The figure shows three views and two pictorial views of one solid part (mm, origin at its lowest corner). Answer the questions. A direction names the side the tool comes from. Give positions to 0.01 mm unless a question says otherwise; leave off trailing zeros. Loops run counter-clockwise (first coordinate to the right, second up) from the corner with the lowest first, then second, coordinate; pieces in that order, holes last. Notation, with made-up numbers: (10, 7.5) -> (65, 7.5) arc R3 ccw to (65, 11.5) -> close; hole circle Ø1 at (71, -15). An arc over 180 degrees is marked (long way). One line per item, written item: value. Start each with the question number.
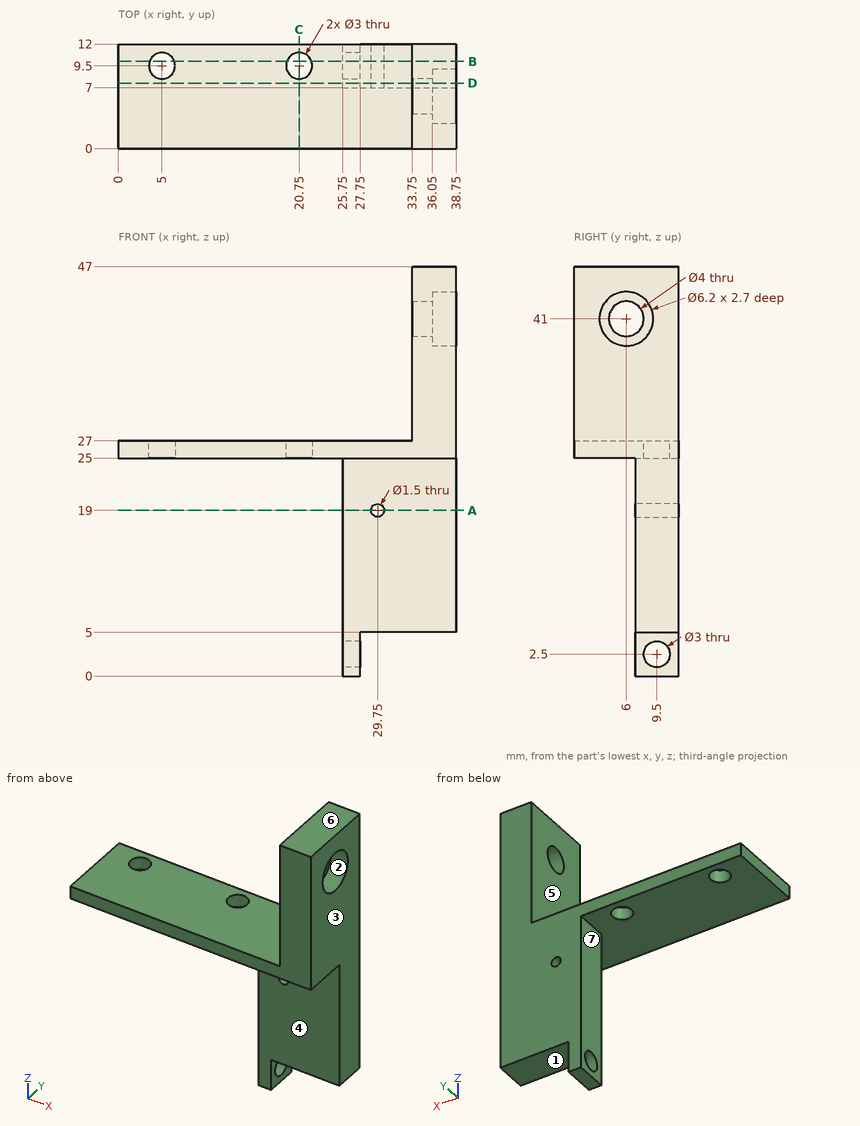
Item 1: Flat-ended cylindrical pins translate along their axes: pin 1 (2.5 mm diameter, centred on x = 29.75, z = 19, fed in from -Y); pin 2 (12 mm diameter, centred on x = 21.5, z = 38, fed in from -Y); pin 3 (1.5 mm diameter, centred on y = 10, z = 1.5, fed in from +X); pin 4 (1.5 mm diameter, centred on y = 9, z = 11, fed in from -X). Find the tip coordinate at first contact, or state that the pin passes through.
Item 2: For the marked faces 4, 5, 6 and 7, determine the directions among +Z, -Z, +X, -X, +Y, -Y from which every point of the face is accessible in a straight line to the end or side of a thin tool.
Item 3: Section D-D, the plane y = 7.5 is taken. Determine the outline of the cut face in (x, z), plus the area to 3 significant figures.
Item 4: Determine the mould class of the marked faces 1, 2 and 3 for opening direction Z: pulls with the +Z half, pulls with the -Z half, needs draft (parallel to the pull), parting line crosses it, or undercut.
Item 5: Consider L1, parallel to X at y = 10.8, z = 19; L2, parallel to Z at x = 37.6, y = 6; L3, parallel to Z at x = 22.5, y = 4.75. Determine where each line is inside the solid, lowest interval first. Write a range as [from, to].
Item 6: Section C-C, the plane x = 20.75 is taken. Determine the outline of the cut face in (y, z).
Item 7: Section A-A, the plane z = 19 is taken. Determine the outline of the cut face in (x, y), plus the area to 3 significant figures.
Item 8: Section B-B, the plane y = 10 is taken. Determine the outline of the cut face in (x, z), plus the area to 3 significant figures.
Computed values:
1. pin 1: y = 7
1. pin 2: through
1. pin 3: x = 27.75
1. pin 4: x = 25.75
2. face 4: -Z, +X, -X, -Y
2. face 5: +Z, -X, +Y, -Y
2. face 6: +Z, +X, -X, +Y, -Y
2. face 7: -Z, -X, +Y, -Y
3. outline: (0, 25) -> (25.75, 25) -> (25.75, 0) -> (27.75, 0) -> (27.75, 5) -> (38.75, 5) -> (38.75, 38.29) -> (36.05, 38.29) -> (36.05, 39.68) -> (33.75, 39.68) -> (33.75, 27) -> (0, 27) -> close; (33.75, 42.32) -> (36.05, 42.32) -> (36.05, 43.71) -> (38.75, 43.71) -> (38.75, 47) -> (33.75, 47) -> close; hole circle Ø1.5 at (29.75, 19)
3. area: 425 mm²
4. face 1: pulls with the -Z half
4. face 2: undercut
4. face 3: needs draft
5. L1: [25.75, 29], [30.5, 38.75]
5. L2: [25, 37.9], [44.1, 47]
5. L3: [25, 27]
6. outline: (0, 25) -> (8, 25) -> (8, 27) -> (0, 27) -> close; (11, 25) -> (12, 25) -> (12, 27) -> (11, 27) -> close
7. outline: (25.75, 7) -> (29, 7) -> (29, 12) -> (25.75, 12) -> close; (30.5, 7) -> (38.75, 7) -> (38.75, 12) -> (30.5, 12) -> close
7. area: 57.5 mm²
8. outline: (0, 25) -> (3.59, 25) -> (3.59, 27) -> (0, 27) -> close; (6.41, 25) -> (19.34, 25) -> (19.34, 27) -> (6.41, 27) -> close; (22.16, 25) -> (25.75, 25) -> (25.75, 3.91) -> (27.75, 3.91) -> (27.75, 5) -> (38.75, 5) -> (38.75, 47) -> (33.75, 47) -> (33.75, 27) -> (22.16, 27) -> close; (25.75, 0) -> (27.75, 0) -> (27.75, 1.09) -> (25.75, 1.09) -> close; hole circle Ø1.5 at (29.75, 19)
8. area: 429 mm²
